from build123d import *

# Parameters (mm, degrees)
EXTRUDE_1_DEPTH      = 32
EXTRUDE_1_DEPTH_BACK = 5
SKETCH_6_W           = 108.75
SKETCH_6_H           = 62.54
SKETCH_8_W           = 100.75
SKETCH_8_H           = 54.54
CUT_EXTRUDE_1_DEPTH  = 7
CUT_EXTRUDE_2_DEPTH  = 23.4
SKETCH_10_W          = 69.18
SKETCH_10_H          = 54.54
CUT_EXTRUDE_3_DEPTH  = 1.6
SKETCH_11_W          = 67.18
SKETCH_11_H          = 52.54
CUT_EXTRUDE_4_DEPTH  = 3
SKETCH_12_W          = 12.2
SKETCH_12_H          = 11
CUT_EXTRUDE_5_DEPTH  = 104.605353144
CUT_EXTRUDE_6_REACH  = 129.537
SKETCH_14_W          = 28.5
SKETCH_14_H          = 4.5
CUT_EXTRUDE_7_REACH  = 103.154
SKETCH_15_W          = 28.41
SKETCH_15_H          = 17.6
EXTRUDE_2_DEPTH      = 5
CUT_EXTRUDE_14_REACH = 129.537
SKETCH_23_W          = 28.5
SKETCH_23_H          = 1.6
SKETCH_25_W          = 104.75
SKETCH_25_H          = 58.54
SKETCH_25_W_2        = 100.75
SKETCH_25_H_2        = 54.54
EXTRUDE_3_DEPTH      = 2
SKETCH_26_W          = 26
SKETCH_26_H          = 13.3
CUT_EXTRUDE_15_DEPTH = 4


with BuildPart() as part:
    # ｽｹｯﾁ6 → ﾎﾞｽ - 押し出し1 (new, two sides: drawn at the far end of the back side and taken through both)
    with BuildSketch(Plane(origin=(0, 0, 0), x_dir=(1, 0, 0), z_dir=(0, 1, 0)).offset(-EXTRUDE_1_DEPTH_BACK)):
        with Locations((18.405, 27.17)):
            Rectangle(SKETCH_6_W, SKETCH_6_H)
    extrude(amount=EXTRUDE_1_DEPTH + EXTRUDE_1_DEPTH_BACK)

    # ｽｹｯﾁ8 → ｶｯﾄ - 押し出し1 (cut)
    with BuildSketch(Plane(origin=(0, 32, 0), x_dir=(1, 0, 0), z_dir=(0, 1, 0))):
        with Locations((18.405, 27.17)):
            Rectangle(SKETCH_8_W, SKETCH_8_H)
    extrude(amount=-CUT_EXTRUDE_1_DEPTH, mode=Mode.SUBTRACT)

    # ｽｹｯﾁ9 → ｶｯﾄ - 押し出し2 (cut)
    with BuildSketch(Plane(origin=(0, 25, 0), x_dir=(1, 0, 0), z_dir=(0, 1, 0))):
        Polygon((-0.5, 54.44), (-0.5, 44.22), (-6.56, 44.22), (-6.56, 32.02), (-0.5, 32.02), (-0.5, 12.82), (-2.06, 12.82), (-2.06, 3.62), (-0.5, 3.62), (-0.5, -0.1), (68.78, -0.1), (68.78, 54.44), align=None)
    extrude(amount=-CUT_EXTRUDE_2_DEPTH, mode=Mode.SUBTRACT)

    # ｽｹｯﾁ10 → ｶｯﾄ - 押し出し3 (cut)
    with BuildSketch(Plane(origin=(0, 1.6, 0), x_dir=(1, 0, 0), z_dir=(0, 1, 0))):
        with Locations((34.09, 27.17)):
            Rectangle(SKETCH_10_W, SKETCH_10_H)
    extrude(amount=-CUT_EXTRUDE_3_DEPTH, mode=Mode.SUBTRACT)

    # ｽｹｯﾁ11 → ｶｯﾄ - 押し出し4 (cut)
    with BuildSketch(Plane(origin=(0, 0, 0), x_dir=(1, 0, 0), z_dir=(0, 1, 0))):
        with Locations((34.09, 27.17)):
            Rectangle(SKETCH_11_W, SKETCH_11_H)
    extrude(amount=-CUT_EXTRUDE_4_DEPTH, mode=Mode.SUBTRACT)

    # ｽｹｯﾁ12 → ｶｯﾄ - 押し出し5 (cut, through all)
    with BuildSketch(Plane(origin=(-6.56, 0, 0), x_dir=(0, 0, -1), z_dir=(1, 0, 0))):
        with Locations((38.12, 7.1)):
            Rectangle(SKETCH_12_W, SKETCH_12_H)
    extrude(amount=-CUT_EXTRUDE_5_DEPTH, mode=Mode.SUBTRACT)

    # ｽｹｯﾁ14 → ｶｯﾄ - 押し出し6 (cut, up to next)
    with BuildSketch(Plane.ZY.offset(35.97), mode=Mode.PRIVATE) as cut_extrude_6_sk1:
        with Locations((-29.97, 16.45)):
            Rectangle(SKETCH_14_W, SKETCH_14_H)
    cut_extrude_6_tool1 = extrude(cut_extrude_6_sk1.sketch, amount=-CUT_EXTRUDE_6_REACH, mode=Mode.PRIVATE) & part.part
    add(cut_extrude_6_tool1.solids().sort_by_distance((-35.97, 16.45, -29.97))[0], mode=Mode.SUBTRACT)

    # ｶｯﾄ - 押し出し7: up to this face of the body (flat: up to its plane)
    cut_extrude_7_end = Plane(part.part.faces().sort_by_distance((18.405, 13.5, -58.44))[0])
    # ｽｹｯﾁ15 → ｶｯﾄ - 押し出し7 (cut, up to the picked face)
    with BuildSketch(Plane.XY.offset(4.1), mode=Mode.PRIVATE) as cut_extrude_7_sk1:
        with Locations((-21.765, 3.8)):
            Rectangle(SKETCH_15_W, SKETCH_15_H)
    cut_extrude_7_tool1 = split(extrude(cut_extrude_7_sk1.sketch, amount=-CUT_EXTRUDE_7_REACH, mode=Mode.PRIVATE), bisect_by=cut_extrude_7_end, keep=Keep.BOTH, mode=Mode.PRIVATE)
    add(cut_extrude_7_tool1.solids().sort_by(Axis((-21.765, 3.8, 4.1), (0, 0, -1)))[0], mode=Mode.SUBTRACT)

    # ｽｹｯﾁ16 → ﾎﾞｽ - 押し出し2 (add)
    with BuildSketch(Plane(origin=(0, 25, 0), x_dir=(1, 0, 0), z_dir=(0, 1, 0))):
        Polygon((-0.5, 54.44), (-31.97, 54.44), (-31.97, -0.1), (0, -0.1), (0, 1.9), (-29.97, 1.9), (-29.97, 52.44), (-0.5, 52.44), align=None)
    extrude(amount=EXTRUDE_2_DEPTH)

    # ｽｹｯﾁ23 → ｶｯﾄ - 押し出し14 (cut, up to next)
    with BuildSketch(Plane.ZY.offset(35.97), mode=Mode.PRIVATE) as cut_extrude_14_sk1:
        with Locations((-29.97, 13.4)):
            Rectangle(SKETCH_23_W, SKETCH_23_H)
    cut_extrude_14_tool1 = extrude(cut_extrude_14_sk1.sketch, amount=-CUT_EXTRUDE_14_REACH, mode=Mode.PRIVATE) & part.part
    add(cut_extrude_14_tool1.solids().sort_by_distance((-35.97, 13.4, -29.97))[0], mode=Mode.SUBTRACT)

    # ｽｹｯﾁ25 → ﾎﾞｽ - 押し出し3 (add)
    with BuildSketch(Plane(origin=(0, 32, 0), x_dir=(1, 0, 0), z_dir=(0, 1, 0))):
        with Locations((18.405, 27.17)):
            Rectangle(SKETCH_25_W, SKETCH_25_H)
        with Locations((18.405, 27.17)):
            Rectangle(SKETCH_25_W_2, SKETCH_25_H_2, mode=Mode.SUBTRACT)
    extrude(amount=EXTRUDE_3_DEPTH)

    # ｽｹｯﾁ26 → ｶｯﾄ - 押し出し15 (cut)
    with BuildSketch(Plane.ZY.offset(-68.78)):
        with Locations((-25.94, 27.35)):
            Rectangle(SKETCH_26_W, SKETCH_26_H)
    extrude(amount=-CUT_EXTRUDE_15_DEPTH, mode=Mode.SUBTRACT)


solid = part.part
Read the model definition and answer for the solid it produces. Units are mm, in the model's axes. A direction names the side the tool comes from. Give positions to 0.01 mm unless a question says otherwise; leave off trailing zeros. Write each loop counter-clockwise with the first axis right and the second up, starting at its lowest first coordinate (ties: lowest second). Pieces come first, ordered by that corner, then holes. Notation, with made-up numbers: (61.25, 31.25) - (80.25, 31.25) arc R17 ccw to (80.25, 55.25) - close; hole circle Ø4 at (-25.5, 14). An arc over 180 degrees is marked (long way). Use CSV: the item, a comma, the result in double quotes. Start each with the question number.
(1) Find section A-A (z = -24.5). Give the vertices of the cut face in (x, y).
(2) Determine the mould class of faces 4 (the flat face through (-22, 12.6, -51)), 5 (the flat face through (0.5, -1, -27)), 6 (the flat face through (-18, 16, -15.72)) for opening direction Y: +Y half, -Y half, draft (parallel to the pull), parting line (faces both ways), or undercut.
(3) Given P1, Ø8, axis at x = -16.5, z = -47.5, coming from the -Y side; P2, Ø1.7, axis at x = -1.5, z = -7, coming from the +Y side; P3, Ø3, axis at y = 16, z = -24, coming from the -X side, each flat-ended and moving along its own axis, determine where each tip first touches the part or whether it passes through.
(4) Find section C-C (z = -45.5). Give the vertices of the cut face in (x, y).
(5) Find section B-B (x = -10). Give the vertices of the cut face in (y, z).
(6) For faces 1 (the flat face through (70.78, 33, -5)), 2 (the flat face through (18, 33, 2.1)), 3 (the flat face through (-30.3, 30, -27.3)), determine the directions among +Z, -Z, +X, -X, +Y, -Y from which every point of the face is accessible in a straight line to the end or side of a thin tool.
(7) Find section D-D (y = 3). Give the vertices of the cut face in (x, z), plus the area to 3 significant figures.
(8) Consider line 1 along X through (y, z) = (18, -45.5); line 2 along X through (y, z) = (23, -7); line 3 along Z through (x, y) = (4.5, 11.5). Determine where each line is inside the solid, lowest interval first.
Findings below:
1,outline,"(-35.97, 18.7) - (-0.5, 18.7) - (-0.5, 25) - (-29.97, 25) - (-29.97, 30) - (-31.97, 30) - (-31.97, 34) - (-33.97, 34) - (-33.97, 32) - (-35.97, 32) - close; (-7.56, -5) - (72.78, -5) - (72.78, 20.7) - (68.78, 20.7) - (68.78, 1.6) - (68.68, 1.6) - (68.68, 0) - (67.68, 0) - (67.68, -3) - (0.5, -3) - (0.5, 0) - (-0.5, 0) - (-0.5, 12.6) - (-7.56, 12.6) - close"
2,face 4,"-Y half"
2,face 5,"draft"
2,face 6,"undercut"
3,P1,"y = 12.6"
3,P2,"y = 25"
3,P3,"x = 68.78"
4,outline,"(-35.97, 12.6) - (-7.56, 12.6) - (-7.56, -5) - (72.78, -5) - (72.78, 32) - (70.78, 32) - (70.78, 34) - (68.78, 34) - (68.78, 1.6) - (68.68, 1.6) - (68.68, 0) - (67.68, 0) - (67.68, -3) - (0.5, -3) - (0.5, 0) - (-0.5, 0) - (-0.5, 25) - (-29.97, 25) - (-29.97, 30) - (-31.97, 30) - (-31.97, 34) - (-33.97, 34) - (-33.97, 32) - (-35.97, 32) - close"
5,outline,"(12.6, -58.44) - (32, -58.44) - (32, -56.44) - (34, -56.44) - (34, -54.44) - (30, -54.44) - (30, -52.44) - (25, -52.44) - (25, -1.9) - (30, -1.9) - (30, 0.1) - (34, 0.1) - (34, 2.1) - (32, 2.1) - (32, 4.1) - (12.6, 4.1) - (12.6, -15.72) - (18.7, -15.72) - (18.7, -44.22) - (12.6, -44.22) - close"
6,face 1,"+Z, -Z, +X, +Y"
6,face 2,"+Z, +X, -X, +Y"
6,face 3,"+Y"
7,outline,"(-7.56, -58.44) - (72.78, -58.44) - (72.78, 4.1) - (-7.56, 4.1) - (-7.56, -32.02) - (-0.5, -32.02) - (-0.5, -12.82) - (-2.06, -12.82) - (-2.06, -3.62) - (-0.5, -3.62) - (-0.5, 0.1) - (68.78, 0.1) - (68.78, -54.44) - (-0.5, -54.44) - (-0.5, -44.22) - (-7.56, -44.22) - close"
7,area,"1,150 mm2"
8,line 1,"-35.97 to -0.5, 68.78 to 72.78"
8,line 2,"-35.97 to -2.06, 68.78 to 72.78"
8,line 3,"-58.44 to -54.44, 0.1 to 4.1"
